Geometry: final body of the model. Coordinates: model frame, mm. Face numbers are marked on the shaded views. A direction names the side the tool comes from. Round coordinates to 2 decimals unless told otherwise and drop trailing zeros. Write each loop counter-clockwise with the first axis right and the second up, starting at its lowest first coordinate (ties: lowest second). Pieces come first, ordered by that corner, then holes. Notation, with made-up numbers: (-27, -32.5) - (5, -32.5) arc R33 cw to (5, 3.5) - close; hole circle Ø5 at (-28, 43). An arc over 180 degrees is marked (long way). Use a Markdown table: item, result. Add a question column.
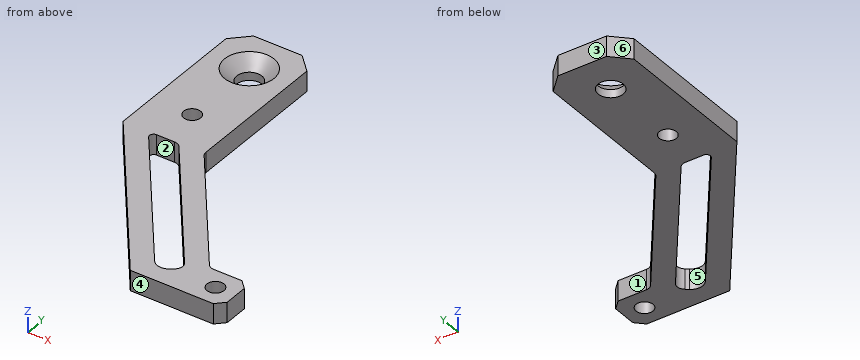
```python
from build123d import *

# Parameters (mm, degrees)
SKETCH_1_R          = 2.1
SKETCH_1_R_2        = 3.1
EXTRUDE_1_DEPTH     = 2.5
FILLET_1_R          = 2
FILLET_2_R          = 3
CHAMFER_1_SIZE      = 4
CHAMFER_2_SIZE      = 2
FILLET_3_R          = 1
SKETCH_2_R          = 2.1
CUT_EXTRUDE_1_DEPTH = 5
CHAMFER_3_SIZE      = 3


with BuildPart() as part:
    # 草图1 → 凸台-拉伸1 (new, symmetric)
    with BuildSketch(Plane.XY):
        Polygon((-10, 10), (-10, -30), (21.776923077, -72.5), (44.3, -72.5), (44.3, -62.5), (34.3, -62.5), (10, -30), (10, 10), align=None)
        with Locations((39.3, -67.5)):
            Circle(SKETCH_1_R, mode=Mode.SUBTRACT)
        Circle(SKETCH_1_R_2, mode=Mode.SUBTRACT)
        Polygon((-3.756916253, -30), (3.756916253, -30), (30.3908691, -65.621541874), (25.686053977, -69.378458126), align=None, mode=Mode.SUBTRACT)
    extrude(amount=EXTRUDE_1_DEPTH, both=True)

    # 圆角1
    fillet_1_edges = [part.edges().sort_by_distance(p)[0] for p in [
        (10, -30, 0),
        (34.3, -62.5, 0),
        (30.3908691, -65.621541874, 0),
        (3.756916253, -30, 0),
    ]]
    fillet(fillet_1_edges, radius=FILLET_1_R)

    # 圆角2
    fillet_2_edges = [part.edges().sort_by_distance(p)[0] for p in [
        (25.686053977, -69.378458126, 0),
    ]]
    fillet(fillet_2_edges, radius=FILLET_2_R)

    # 倒角1
    chamfer_1_edges = [part.edges().sort_by_distance(p)[0] for p in [
        (10, 10, 0),
        (-10, 10, 0),
    ]]
    chamfer(chamfer_1_edges, length=CHAMFER_1_SIZE)

    # 倒角2
    chamfer_2_edges = [part.edges().sort_by_distance(p)[0] for p in [
        (44.3, -62.5, 0),
        (44.3, -72.5, 0),
    ]]
    chamfer(chamfer_2_edges, length=CHAMFER_2_SIZE)

    # 圆角3
    fillet_3_edges = [part.edges().sort_by_distance(p)[0] for p in [
        (-3.756916253, -30, 0),
    ]]
    fillet(fillet_3_edges, radius=FILLET_3_R)

    # 草图2 → 切除-拉伸1 (cut)
    with BuildSketch(Plane.XY.offset(2.5)):
        with Locations((0, -20)):
            Circle(SKETCH_2_R)
    extrude(amount=-CUT_EXTRUDE_1_DEPTH, mode=Mode.SUBTRACT)

    # 倒角3
    chamfer_3_edges = [part.edges().sort_by_distance(p)[0] for p in [
        (-3.1, 0, 2.5),
    ]]
    chamfer(chamfer_3_edges, length=CHAMFER_3_SIZE)


solid = part.part
```
1) Pin query (flat end, axial travel): P1, Ø2, axis at y = -32, z = 1, coming from the +X side; P2, Ø1.5, axis at y = -6.5, z = 1, coming from the +X side; P3, Ø7, axis at x = 0, y = 0, coming from the +Z side. Return the tip coordinate at first contact, or that it passes through.
2) Set-up query: the marked faces 1, 2 and 3. Return all of +Z, -Z, +X, -X, +Y, -Y with unobstructed straight access to the full face (end or side cutting, diameter ignored); none if empty.
3) Section C-C, the plane x = 39.3. Return the cut outline in (y, z).
4) Section B-B, the plane z = 0.4. Return the cut outline in (x, y).
5) Section D-D, the plane x = 0. Return the cut outline in (y, z), then the cut area to 3 significant figures.
6) Draft query along X for the marked faces 4, 5 and 6. Return one class per face: released by +X, released by -X, zero draft, split by the parting line, or undercut.
7) Section A-A, the plane y = -20. Return the cut outline in (x, z).
8) Material intervals for L1, parallel to X at y = -66, z = 1.4; L2, parallel to Y at x = 0, z = -1.1; L3, parallel to Y at x = 41.5, z = -0.65, sorted ascending. Write a range as from..to.
Output values:
| question | item | result |
|---|---|---|
| 1 | P1 | stops at x = 12.24 |
| 1 | P2 | stops at x = 10 |
| 1 | P3 | stops at z = -0.1 |
| 2 | face 1 | +Z, -Z, +X, +Y |
| 2 | face 2 | +Z, -Z |
| 2 | face 3 | +Z, -Z, +X, -X, +Y |
| 3 | outline | (-72.5, -2.5) - (-69.6, -2.5) - (-69.6, 2.5) - (-72.5, 2.5) - close; (-65.4, -2.5) - (-62.5, -2.5) - (-62.5, 2.5) - (-65.4, 2.5) - close |
| 4 | outline | (-10, -30) - (21.78, -72.5) - (42.3, -72.5) - (44.3, -70.5) - (44.3, -64.5) - (42.3, -62.5) - (35.3, -62.5) arc R2 cw to (33.7, -61.7) - (10.4, -30.53) arc R2 cw to (10, -29.33) - (10, 6) - (6, 10) - (-6, 10) - (-10, 6) - close; hole circle Ø8 at (0, 0); hole (-2.56, -31.6) - (23.83, -66.9) arc R3 ccw to (28.11, -67.45) - (28.88, -66.83) arc R2 ccw to (29.23, -64.07) - (4.36, -30.8) arc R2 ccw to (2.76, -30) - (-1.76, -30) arc R1 ccw to start; hole circle Ø4.2 at (0, -20); hole circle Ø4.2 at (39.3, -67.5) |
| 5 | outline | (-43.37, -2.5) - (-35.02, -2.5) - (-35.02, 2.5) - (-43.37, 2.5) - close; (-30, -2.5) - (-22.1, -2.5) - (-22.1, 2.5) - (-30, 2.5) - close; (-17.9, -2.5) - (-3.1, -2.5) - (-3.1, -0.5) - (-6.1, 2.5) - (-17.9, 2.5) - close; (3.1, -2.5) - (10, -2.5) - (10, 2.5) - (6.1, 2.5) - (3.1, -0.5) - close |
| 5 | area | 181 mm^2 |
| 6 | face 4 | zero draft |
| 6 | face 5 | undercut |
| 6 | face 6 | released by -X |
| 7 | outline | (-10, -2.5) - (-2.1, -2.5) - (-2.1, 2.5) - (-10, 2.5) - close; (2.1, -2.5) - (10, -2.5) - (10, 2.5) - (2.1, 2.5) - close |
| 8 | L1 | x = 16.92..23.16, 29.49..37.83, 40.77..44.3 |
| 8 | L2 | y = -43.37..-35.02, -30..-22.1, -17.9..-3.1, 3.1..10 |
| 8 | L3 | y = -72.5..-62.5 |
